Verification items for the finished model (mm, model axes). A direction names the side the tool comes from. Coordinates: 2 decimals unless noted, no trailing zeros. Loops run counter-clockwise (first coordinate to the right, second up) from the corner with the lowest first, then second, coordinate; pieces in that order, holes last.
Q1. Sectioned sample at C-C (z = -24). Enter the section's corners in (x, y).
Q2. Sectioned sample at B-B (y = 10.5). Enter the section's corners in (x, z), then the cut area to 4 significant figures.
Q3. Sectioned sample at D-D (x = 19). Enter the section's corners in (y, z).
Q4. Go/stop test with flat-tipped pins: P1, Ø3, axis at x = 3, z = -18, coming from the +Y side; P2, Ø18.5, axis at x = 21, z = -23.5, coming from the -Y side; P3, Ø3, axis at x = 31, y = 18, coming from the +Z side. Record where each tip stops, or that it passes through.
Q5. Sectioned sample at A-A (y = 4). Enter the section's corners in (x, z).
Q6. Material ranges on probe 1 along Z at (x, y) = (31, 6.5); probe 2 along X at (y, z) = (1, -19.5); probe 3 along Y at (x, z) = (11, -38), recorded low to high.
Q7. Access from +Z, -Z, +X, -X, +Y, -Y to the whole of each face (thin tool, end or side, straight path). Record for faces 1 (the face through (3, 0.1, -30.5)), 2 (the face through (3, 28, -20)), 3 (the face through (32, 16, -5)), 4 (the face through (32, 16, -36)).
Q8. Mould release check, pull along X, two halves, no side actions. Record for faces 5 (the face through (32.444, 0.07, -10.769)), 6 (the face through (32, 28, -20)): +X half, -X half, draft (parallel to the pull), parting line (faces both ways), or undercut.
```python
from build123d import *

# Parameters (mm, degrees)
SKETCH_1_W          = 35
SKETCH_1_H          = 41
EXTRUDE_1_DEPTH     = 33
SKETCH_3_W          = 41
SKETCH_3_H          = 33
SKETCH_3_W_2        = 31
SKETCH_3_H_2        = 23
CUT_EXTRUDE_1_DEPTH = 6
SKETCH_2_R          = 0.5
EXTRUDE_2_DEPTH     = 10


with BuildPart() as part:
    # 草图1 → 凸台-拉伸1 (new body)
    with BuildSketch(Plane(origin=(0, 0, 0), x_dir=(1, 0, 0), z_dir=(0, 1, 0))):
        with Locations((17.5, 20.5)):
            Rectangle(SKETCH_1_W, SKETCH_1_H)
    extrude(amount=EXTRUDE_1_DEPTH)

    # 草图3 → 切除-拉伸1 (cut)
    with BuildSketch(Plane(origin=(35, 0, 0), x_dir=(0, 0, -1), z_dir=(1, 0, 0))):
        with Locations((20.5, 16.5)):
            Rectangle(SKETCH_3_W, SKETCH_3_H)
        with Locations((20.5, 16.5)):
            Rectangle(SKETCH_3_W_2, SKETCH_3_H_2, mode=Mode.SUBTRACT)
    cut_extrude_1 = extrude(amount=-CUT_EXTRUDE_1_DEPTH, mode=Mode.SUBTRACT)

    # 镜向9: 切除-拉伸1 across plane
    add(cut_extrude_1.mirror(Plane(origin=(17.5, 0, 0), x_dir=(0, 0, 1), z_dir=(1, 0, 0))), mode=Mode.SUBTRACT)

    # 草图2 → 凸台-拉伸2 (add)
    with BuildSketch(Plane.XZ.offset(-5)):
        with Locations(Location((3, -11, 0), (0, 0, 90))):
            Circle(SKETCH_2_R)
        with Locations(Location((3, -30, 0), (0, 0, 90))):
            Circle(SKETCH_2_R)
        with Locations(Location((32, -30, 0), (0, 0, 270))):
            Circle(SKETCH_2_R)
        with Locations(Location((32, -11, 0), (0, 0, 90))):
            Circle(SKETCH_2_R)
        with Locations(Location((32, -20.5, 0), (0, 0, 90))):
            Circle(SKETCH_2_R)
    extrude(amount=EXTRUDE_2_DEPTH)


solid = part.part
```
Geometry check:
1. outline: (0, 5) - (6, 5) - (6, 0) - (29, 0) - (29, 5) - (35, 5) - (35, 28) - (29, 28) - (29, 33) - (6, 33) - (6, 28) - (0, 28) - close
2. outline: (0, -36) - (6, -36) - (6, -41) - (29, -41) - (29, -36) - (35, -36) - (35, -5) - (29, -5) - (29, 0) - (6, 0) - (6, -5) - (0, -5) - close
2. area: 1,315 mm2
3. outline: (0, -41) - (33, -41) - (33, 0) - (0, 0) - close
4. P1: stops at y = 28
4. P2: stops at y = 0
4. P3: stops at z = -5
5. outline: circle Ø1 at (3, -30); circle Ø1 at (3, -11); (6, -41) - (29, -41) - (29, 0) - (6, 0) - close; circle Ø1 at (32, -30); circle Ø1 at (32, -20.5); circle Ø1 at (32, -11)
6. probe 1: z = -36 to -5
6. probe 2: x = 6 to 29
6. probe 3: y = 0 to 33
7. face 1: -Y
7. face 2: +Z, -Z, -X, +Y
7. face 3: +Z, +X, +Y, -Y
7. face 4: -Z, +X, +Y, -Y
8. face 5: undercut
8. face 6: draft
